Source: three-view drawing plus pictorial views. Frame: mm from the lowest corner of the part. Give positions to 0.01 mm unless a question says otherwise; leave off trailing zeros. Write each loop counter-clockwise with the first axis right and the second up, starting at its lowest first coordinate (ties: lowest second). Pieces come first, ordered by that corner, then holes. Notation, with made-up numbers: (47.5, 82.25) - (57.5, 82.25) arc R14 ccw to (57.5, 94.25) - close; hole circle Ø10 at (88, 79.5). An arc over 180 degrees is marked (long way). One line per question, with ' | ' between items. Start each with the question number.
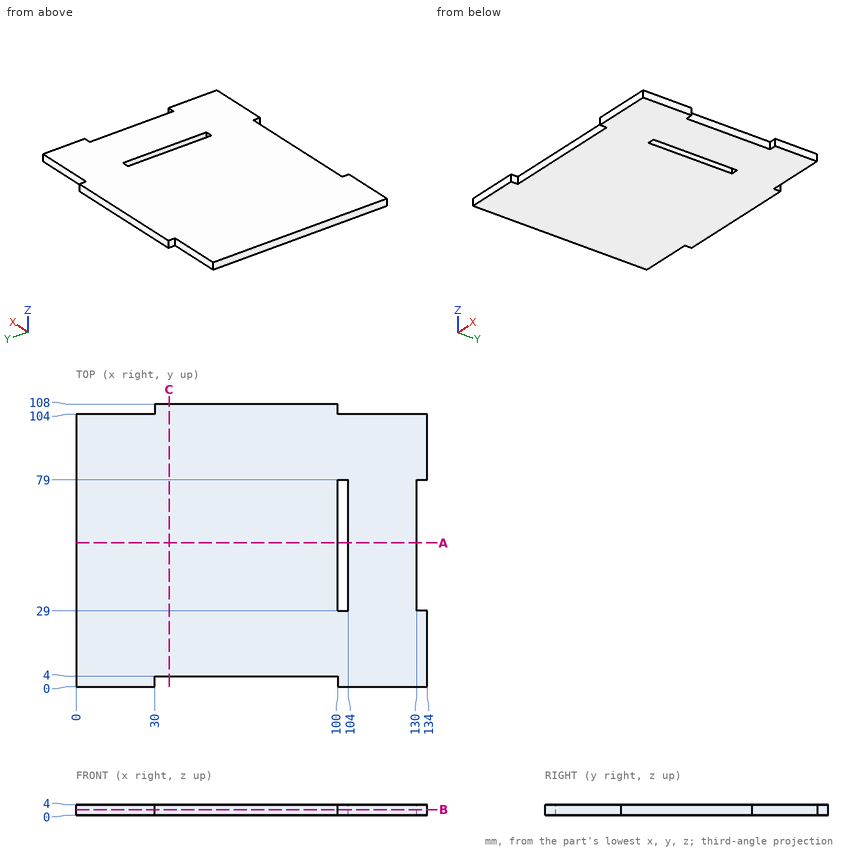
1) Line query: L1, parallel to X at y = 70.5, z = 0.85; L2, parallel to Y at x = 18, z = 1.4; L3, parallel to Y at x = 34.5, z = 3.2. Output: solid intervals per line, ascending.
2) Section C-C, the plane x = 35.5. Output: boundary loops of the cut face in (y, z).
3) First-contact query: pin 1 Ø2 at (x, z) = (132, 1.5) entering from +Y; pin 2 Ø1 at (y, z) = (76.5, 3) entering from +X. Flat tips, straight axial feed; report the tip coordinate or a pass-through.
4) Section B-B, the plane z = 2.25. Output: boundary loops of the cut face in (x, y).
5) Section A-A, the plane y = 55. Output: boundary loops of the cut face in (x, z).
Answer key:
1) L1: 0 to 100, 104 to 130 | L2: 0 to 104 | L3: 4 to 108
2) outline: (4, 0) - (108, 0) - (108, 4) - (4, 4) - close
3) pin 1: y = 104 | pin 2: x = 130
4) outline: (0, 0) - (30, 0) - (30, 4) - (100, 4) - (100, 0) - (134, 0) - (134, 29) - (130, 29) - (130, 79) - (134, 79) - (134, 104) - (100, 104) - (100, 108) - (30, 108) - (30, 104) - (0, 104) - close; hole (100, 29) - (104, 29) - (104, 79) - (100, 79) - close
5) outline: (0, 0) - (100, 0) - (100, 4) - (0, 4) - close; (104, 0) - (130, 0) - (130, 4) - (104, 4) - close
